Geometry check sheet. Reference: the model listing, model coordinates, mm. A direction names the side the tool comes from. Round coordinates to 2 decimals unless told otherwise and drop trailing zeros. Order: outer loops, then holes, each group sorted by start corner. A loop starts at its lowest first (then second) coordinate and runs counter-clockwise, first axis right, second up.
(1) Material ranges on line 1 along X through (y, z) = (-0.25, 5.5); line 2 along Z through (x, y) = (-1.25, 1); line 3 along Y through (x, z) = (3, 7.6), recorded low to high.
(2) Sectioned sample at C-C (z = 5.75). Record the boundary of the cut face in (x, y) (3 decimals).
(3) Set-up check for faces 1 (the face through (0, 0, 0)), 2 (the face through (-3.596, -2.685, 7.521)): record each of +Z, -Z, +X, -X, +Y, -Y from which the full face is reachable in a straight line by a thin tool's end or side.
(4) Sectioned sample at A-A (y = 0). Record the boundary of the cut face in (x, z) (3 decimals).
(5) Go/stop test with flat-tipped pins: pin 1 (3.5 mm diameter, centred on x = -3, y = 0, fed in from -Z); pin 2 (3 mm diameter, centred on x = -4, z = 8, fed in from -Y); pin 3 (3 mm diameter, centred on x = 2, y = 0.5, fed in from +Z). Record where each tip stops, or that it passes through.
(6) Release check for a two-part mould opening along Y. For faces 3 (the face through (-3, -2, 6)), 4 (the face through (3.45, -6.63, 4.94)), 5 (the face through (0, 0, 9)) record: +Y half, -Y half, draft (parallel to the pull), parting line (faces both ways), or undercut.
from build123d import *

# Parameters (mm, degrees)
SKETCH1_R           = 7.5
BOSS_EXTRUDE1_DEPTH = 1
SKETCH2_R           = 7.475
BOSS_EXTRUDE2_DEPTH = 8
SKETCH3_R           = 1.55
CUT_EXTRUDE1_DEPTH  = 14.910427743
SKETCH4_R           = 2.75
CUT_EXTRUDE2_DEPTH  = 3


with BuildPart() as part:
    # Sketch1 → Boss-Extrude1 (new body)
    with BuildSketch(Plane.XY):
        Circle(SKETCH1_R)
    extrude(amount=BOSS_EXTRUDE1_DEPTH)

    # Sketch2 → Boss-Extrude2 (add)
    with BuildSketch(Plane.XY.offset(1)):
        Circle(SKETCH2_R)
    extrude(amount=BOSS_EXTRUDE2_DEPTH)

    # Sketch3 → Cut-Extrude1 (cut, through all)
    with BuildSketch(Plane.XY.offset(9)):
        with Locations((-3, 0)):
            Circle(SKETCH3_R)
        with Locations(Location((3, 0, 0), (0, 0, 180))):
            Circle(SKETCH3_R)
    extrude(amount=-CUT_EXTRUDE1_DEPTH, mode=Mode.SUBTRACT)

    # Sketch4 → Cut-Extrude2 (cut)
    with BuildSketch(Plane.XY.offset(9)):
        with Locations((-3, 0)):
            Circle(SKETCH4_R)
        with Locations(Location((3, 0, 0), (0, 0, 180))):
            Circle(SKETCH4_R)
    extrude(amount=-CUT_EXTRUDE2_DEPTH, mode=Mode.SUBTRACT)


solid = part.part
Answer below:
1. line 1: x = -7.47 to -4.53, -1.47 to 1.47, 4.53 to 7.47
1. line 2: z = 0 to 6
1. line 3: y = -6.85 to -2.75, 2.75 to 6.85
2. outline: circle Ø14.95 at (0, 0); hole circle Ø3.1 at (-3, 0); hole circle Ø3.1 at (3, 0)
3. face 1: -Z, +X, -X, +Y, -Y
3. face 2: +Z
4. outline: (-7.5, 0) - (-4.55, 0) - (-4.55, 6) - (-5.75, 6) - (-5.75, 9) - (-7.475, 9) - (-7.475, 1) - (-7.5, 1) - close; (-1.45, 0) - (1.45, 0) - (1.45, 6) - (0.25, 6) - (0.25, 9) - (-0.25, 9) - (-0.25, 6) - (-1.45, 6) - close; (4.55, 0) - (7.5, 0) - (7.5, 1) - (7.475, 1) - (7.475, 9) - (5.75, 9) - (5.75, 6) - (4.55, 6) - close
5. pin 1: stops at z = 0
5. pin 2: stops at y = -7.04
5. pin 3: stops at z = 6
6. face 3: undercut
6. face 4: parting line
6. face 5: draft
